Can you work these out from the model? Positions are in its coordinate system, mm. Face numbers are marked on the shaded views. A direction names the side the tool comes from. Coordinates: 2 decimals unless noted, no trailing zeros. Order: outer loops, then holes, each group sorted by start corner. A loop starts at its lowest first (then second) coordinate and runs counter-clockwise, first axis right, second up. Notation, with made-up numbers: (66, -27.5) -> (121, -27.5) arc R13 cw to (121, -6.5) -> close; hole circle Ø1 at (78.25, 61.25). An arc over 180 degrees is marked (long way). Answer in a Markdown table with one row per item. Add a question column.
1. We'd pull the mould along X, two halves only. Please class the marked faces 5, 6 and 7: pulls with the +X half, pulls with the -X half, needs draft (parallel to the pull), parting line crosses it, or undercut.
2. If I drill on line 1 along Y through (x, z) = (0, 4); line 2 along Z through (x, y) = (-5, -2.5); line 3 along X through (y, z) = (0.25, 13), over which ranges is the centre line in solid material (lowest first)? Write a range as [from, to].
3. Imagine slicing it at D-D on x = -28. Write out the boundary of the cut face in (y, z), plus the area to 3 significant figures.
4. Imagine slicing it at A-A on y = 0. Write out the boundary of the cut face in (x, z), plus the area to 3 significant figures.
5. Will these pins go through, and if not, where does the flat tip stop? pin 1 (4 mm diameter, centred on x = -24, z = 6.5, fed in from +Y); pin 2 (2.5 mm diameter, centred on x = 14.5, y = -19.5, fed in from +Z); pin 3 (10 mm diameter, centred on x = -29.5, z = 12, fed in from -Y); pin 4 (7 mm diameter, centred on x = 0, y = 0, fed in from +Z).
6. On a 3-axis mill with a long thin cutter (end or side, diameter ignored), from which of +Z, -Z, +X, -X, +Y, -Y can I reach the whole of each face in a straight line? I mean the marked faces 1, 2, 3 and 4. Say none if no direction works.
7. Imagine slicing it at C-C on x = 0. Write out the boundary of the cut face in (y, z).
8. Imagine slicing it at B-B on z = 3. Write out the boundary of the cut face in (x, y), plus the area to 3 significant figures.
from build123d import *

# Parameters (mm, degrees)
SKETCH2_R           = 4
BOSS_EXTRUDE1_DEPTH = 20
SKETCH3_R           = 7.5
BOSS_EXTRUDE2_DEPTH = 36
BOSS_EXTRUDE3_START = -20
BOSS_EXTRUDE3_DEPTH = 20
CUT_EXTRUDE1_DEPTH  = 2
CUT_EXTRUDE2_REACH  = 83.026
BOSS_EXTRUDE4_DEPTH = 2


with BuildPart() as part:
    # Sketch2 → Boss-Extrude1 (new body)
    with BuildSketch(Plane.XY):
        with BuildLine():
            Line((-67.162602834, 1.5), (-6.837397166, 1.5))
            ThreePointArc((-6.837397166, 1.5), (7, 0), (-6.837397166, -1.5))
            Line((-6.837397166, -1.5), (-67.162602834, -1.5))
            Line((-67.162602834, -1.5), (-67.162602834, 1.5))
        make_face()
        Circle(SKETCH2_R, mode=Mode.SUBTRACT)
    extrude(amount=BOSS_EXTRUDE1_DEPTH)

    # Sketch3 → Boss-Extrude2 (add)
    with BuildSketch(Plane.XY.offset(20)):
        with Locations((-67.162602834, 0)):
            Circle(SKETCH3_R)
    extrude(amount=-BOSS_EXTRUDE2_DEPTH)

    # Sketch4 → Boss-Extrude3 (add)
    with BuildSketch(Plane.XY.offset(20).offset(BOSS_EXTRUDE3_START)):
        with BuildLine():
            Line((15.158562953, -19.905224671), (13.520258864, -21.052377544))
            Line((13.520258864, -21.052377544), (3.154702075, -6.248828276))
            ThreePointArc((3.154702075, -6.248828276), (4.015035054, -5.73406431), (4.793006163, -5.101675403))
            Line((4.793006163, -5.101675403), (15.158562953, -19.905224671))
        make_face()
    extrude(amount=BOSS_EXTRUDE3_DEPTH)

    # Sketch5 → Cut-Extrude1 (cut)
    with BuildSketch(Plane(origin=(0.8191520442889967, 0.5735764363510467, 0), x_dir=(0, 0, -1), z_dir=(0.8191520442889931, 0.5735764363510442, 0))):
        with BuildLine():
            Line((-11, -22.346237219), (-11, -25))
            Line((-11, -25), (-9, -25))
            Line((-9, -25), (-9, -22.346237219))
            ThreePointArc((-9, -22.346237219), (-10, -19.72820323), (-11, -22.346237219))
        make_face()
    extrude(amount=-CUT_EXTRUDE1_DEPTH, mode=Mode.SUBTRACT)

    # Sketch6 → Cut-Extrude2 (cut, up to next)
    with BuildSketch(Plane(origin=(0.8191520442889967, 0.5735764363510467, 0), x_dir=(0, 0, -1), z_dir=(0.8191520442889931, 0.5735764363510442, 0)), mode=Mode.PRIVATE) as cut_extrude2_sk1:
        Polygon((-20, -6.92820323), (-15.5, -25), (-21.37977423, -25), (-21.37977423, -6.621098629), align=None)
    cut_extrude2_tool1 = extrude(cut_extrude2_sk1.sketch, amount=-CUT_EXTRUDE2_REACH, mode=Mode.PRIVATE) & part.part
    # Sketch6 → Cut-Extrude2 (cut, up to next)
    with BuildSketch(Plane(origin=(0.8191520442889967, 0.5735764363510467, 0), x_dir=(0, 0, -1), z_dir=(0.8191520442889931, 0.5735764363510442, 0)), mode=Mode.PRIVATE) as cut_extrude2_sk2:
        Polygon((0, -6.92820323), (1.41409792, -6.92820323), (1.41409792, -25), (-4.5, -25), align=None)
    cut_extrude2_tool2 = extrude(cut_extrude2_sk2.sketch, amount=-CUT_EXTRUDE2_REACH, mode=Mode.PRIVATE) & part.part
    add(cut_extrude2_tool1.solids().sort_by_distance((11.026351, -14.003814, 19.337545))[0], mode=Mode.SUBTRACT)
    add(cut_extrude2_tool2.solids().sort_by_distance((11.036642, -14.018511, 0.648226))[0], mode=Mode.SUBTRACT)

    # Sketch7 → Boss-Extrude4 (add)
    with BuildSketch(Plane.XY.offset(9)):
        Polygon((-25.248427633, -1.5), (8.33748047, -13.65060291), (3.154702075, -6.248828276), (-6.837397166, -1.5), align=None)
    extrude(amount=BOSS_EXTRUDE4_DEPTH)


solid = part.part
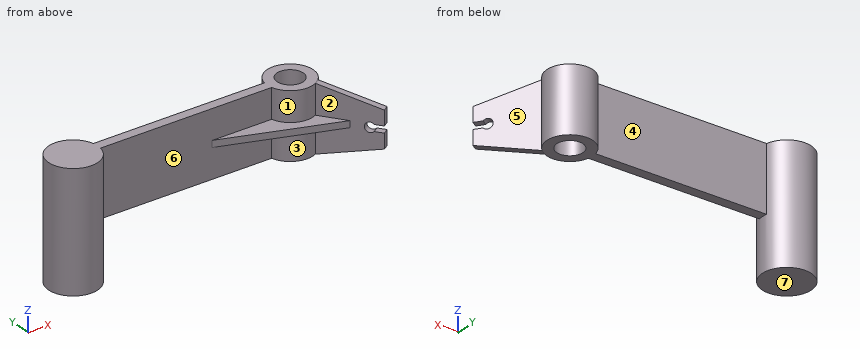
Answers follow:
| question | item | result |
|---|---|---|
| 1 | face 5 | pulls with the +X half |
| 1 | face 6 | undercut |
| 1 | face 7 | needs draft |
| 2 | line 1 | y = [-7, -4], [4, 7] |
| 2 | line 2 | z = [0, 20] |
| 2 | line 3 | x = [-74.66, -3.99], [3.99, 7] |
| 3 | outline | (-1.5, 0) -> (1.5, 0) -> (1.5, 20) -> (-1.5, 20) -> close |
| 3 | area | 60.0 mm² |
| 4 | outline | (-74.66, -16) -> (-59.66, -16) -> (-59.66, 0) -> (-4, 0) -> (-4, 20) -> (-74.66, 20) -> close; (4, 0) -> (7, 0) -> (7, 20) -> (4, 20) -> close |
| 4 | area | 1,710 mm² |
| 5 | pin 1 | stops at y = 1.5 |
| 5 | pin 2 | stops at z = 15.99 |
| 5 | pin 3 | stops at y = -1.73 |
| 5 | pin 4 | passes through |
| 6 | face 1 | +Z, -Y |
| 6 | face 2 | -Y |
| 6 | face 3 | -Z, -Y |
| 6 | face 4 | +Z, -Z, +Y |
| 7 | outline | (-10.63, 9) -> (-7, 9) -> (-7, 0) -> (-4, 0) -> (-4, 20) -> (-7, 20) -> (-7, 11) -> (-10.63, 11) -> close; (4, 0) -> (7, 0) -> (7, 20) -> (4, 20) -> close |
| 8 | outline | (-59.81, -1.5) -> (-6.84, -1.5) arc R7 ccw to (3.15, -6.25) -> (10.07, -16.12) -> (11.7, -14.97) -> (4.79, -5.1) arc R7 ccw (long way) to (-6.84, 1.5) -> (-59.81, 1.5) arc R7.5 ccw (long way) to start; hole circle Ø8 at (0, 0) |
| 8 | area | 463 mm² |
